Job drawing, mm, ordinate dimensions from the low corner. One solid piece. Give positions to 0.01 mm unless a question says otherwise; leave off trailing zeros. Write each loop counter-clockwise with the first axis right and the second up, starting at its lowest first coordinate (ties: lowest second). Pieces come first, ordered by that corner, then holes. Notation, with made-up numbers: (85.25, 45) -> (108.25, 45) arc R21 ccw to (108.25, 51) -> close; hole circle Ø2 at (56, 81). An arc over 180 degrees is marked (long way). One line per question, with ' | ' between items. Start each with the question number.
(1) Band-saw the part on B-B, the plane y = 1.75. Give the cut face in (x, z).
(2) Drill centre lines: probe 1 along Z at (x, y) = (62.5, 2.75); probe 2 along X at (y, z) = (7, 23.5); probe 3 along Y at (x, z) = (6, 35). Where is each one in solid material? Low to high. Write a range as from..to.
(3) Band-saw the part on D-D, the plane x = 2.5. Give the cut face in (y, z), and give its area (3 significant figures).
(4) Band-saw the part on A-A, the plane z = 11.5. Give the cut face in (x, y).
(5) Band-saw the part on C-C, the plane z = 3.5. Give the cut face in (x, y).
(6) Pull direction X, two halves, no side cores. Call the marked faces 1, 2, 3 and 4: released by +X, released by -X, zero draft, split by the parting line, or undercut.
(7) Pin check, flat tips, straight feed: P1, Ø2.5, axis at x = 5, y = 2.5, coming from the -Z side; P2, Ø2, axis at x = 30.5, z = 4.5, coming from the -Y side; P3, Ø2, axis at y = 3, z = 21.5, coming from the +X side; P4, Ø3.5, axis at x = 38.5, y = 6.5, coming from the +Z side. Stop position of each tip, or through.
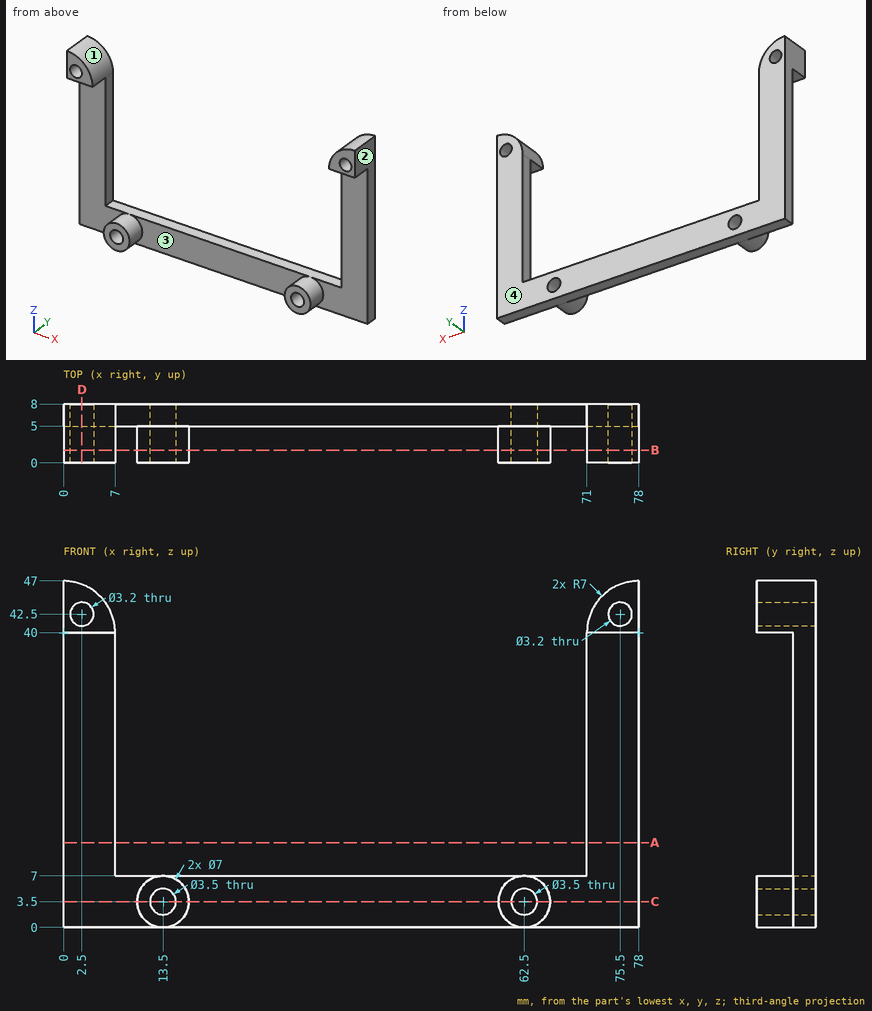
Results:
1) outline: (0, 40) -> (7, 40) arc R7 ccw to (0, 47) -> close; circle Ø7 at (13.5, 3.5); circle Ø7 at (62.5, 3.5); (71, 40) -> (78, 40) -> (78, 47) arc R7 ccw to start; hole circle Ø3.2 at (2.5, 42.5); hole circle Ø3.5 at (13.5, 3.5); hole circle Ø3.5 at (62.5, 3.5); hole circle Ø3.2 at (75.5, 42.5)
2) probe 1: z = 0..1.75, 5.25..7 | probe 2: x = 0..7, 71..78 | probe 3: y = 5..8
3) outline: (0, 40) -> (5, 40) -> (5, 0) -> (8, 0) -> (8, 40.9) -> (0, 40.9) -> close; (0, 44.1) -> (8, 44.1) -> (8, 46.54) -> (0, 46.54) -> close | area: 147 mm²
4) outline: (0, 5) -> (7, 5) -> (7, 8) -> (0, 8) -> close; (71, 5) -> (78, 5) -> (78, 8) -> (71, 8) -> close
5) outline: (0, 5) -> (10, 5) -> (10, 0) -> (11.75, 0) -> (11.75, 8) -> (0, 8) -> close; (15.25, 0) -> (17, 0) -> (17, 5) -> (59, 5) -> (59, 0) -> (60.75, 0) -> (60.75, 8) -> (15.25, 8) -> close; (64.25, 0) -> (66, 0) -> (66, 5) -> (78, 5) -> (78, 8) -> (64.25, 8) -> close
6) face 1: undercut | face 2: released by +X | face 3: undercut | face 4: zero draft
7) P1: stops at z = 40 | P2: stops at y = 5 | P3: passes through | P4: stops at z = 7
